from build123d import *

# Parameters (mm, degrees)
F0_W     = 72
F0_H     = 45
F1_DEPTH = 30
F3_DEPTH = 18
F4_R     = 2
F5_DEPTH = 19
F6_R     = 1.5
F7_R     = 3


with BuildPart() as f1:
    # F0 (on Front) → F1 (new body)
    with BuildSketch(Plane.XZ):
        with Locations((-36, 0)):
            Rectangle(F0_W, F0_H)
    extrude(amount=-F1_DEPTH)

    # F2 (on face) → F3 (join)
    with BuildSketch(Plane.XZ):
        Polygon((-64, 10.8), (-64, -10.8), (-57.15, -17.65), (-50.3, -10.8), (-50.3, 10.8), (-57.15, 17.65), align=None)
    extrude(amount=F3_DEPTH)

    # F4 (on face) → F5 (join)
    with BuildSketch(Plane.XZ.offset(18)):
        with Locations((-57.15, 9.3)):
            Circle(F4_R)
        with Locations((-57.15, -9.3)):
            Circle(F4_R)
    extrude(amount=F5_DEPTH)

    # F6
    f6_edges = [f1.edges().sort_by_distance(p)[0] for p in [
        (-59.15, -37, 9.3),
        (-59.15, -37, -9.3),
    ]]
    fillet(f6_edges, radius=F6_R)

    # F7
    f7_edges = [f1.edges().sort_by_distance(p)[0] for p in [
        (-72, 15, 22.5),
        (-72, 15, -22.5),
        (-72, 0, 0),
        (-72, 30, 0),
        (0, 15, -22.5),
        (0, 15, 22.5),
        (0, 0, 0),
        (0, 30, 0),
        (-36, 0, 22.5),
        (-36, 30, 22.5),
        (-36, 0, -22.5),
        (-36, 30, -22.5),
    ]]
    fillet(f7_edges, radius=F7_R)


solid = f1.part
Work out the finished part from the listing and answer in its coordinate system (mm). A direction names the side the tool comes from. Give positions to 0.01 mm unless a question says otherwise; leave off trailing zeros. Order: outer loops, then holes, each group sorted by start corner. A loop starts at its lowest first (then second) coordinate and runs counter-clockwise, first axis right, second up. Notation, with made-up numbers: (86, 10.5) - (101, 10.5) arc R22 ccw to (101, 40.5) - close; hole circle Ø4 at (63.25, 60). An arc over 180 degrees is marked (long way). Answer as CSV lines item,"result". Start each with the question number.
Q1. The mould has two halves that part along Z. Classify faces 5 (the face through (-59.148, -26.627, -9.212)), 6 (the face through (-57, -18, 0)), 7 (the face through (-36, 15, -22.5)), 8 (the face through (-64, -9, 0)): +Z half, -Z half, draft (parallel to the pull), parting line (faces both ways), or undercut.
Q2. Given pin 1 Ø5.5 at (y, z) = (-12, 1.5) entering from -X; pin 2 Ø3 at (y, z) = (-15.5, -16.5) entering from +X; pin 3 Ø12 at (y, z) = (-2, -4.5) entering from -X; pin 4 Ø8 at (y, z) = (-28.5, -13.5) entering from +X, each flat-ended and moving along its own axis, determine where each tip first touches the part or whether it passes through.
Q3. For faces 1 (the face through (-53.8, -8.9, -14.3)), 2 (the face through (-59.148, -26.627, 9.388)), 3 (the face through (-50.3, -9, 0)), 4 (the face through (-60.5, -8.9, 14.3)), determine the directions among +Z, -Z, +X, -X, +Y, -Y from which every point of the face is accessible in a straight line to the end or side of a thin tool.
Q4. Find the intervals of material crossed by L1, parallel to Y at x = -24.5, z = 1.5; L2, parallel to X at y = -8, z = -1.5; L3, parallel to Y at x = -62, z = 4, in increasing order. Write a range as [from, to].
Q5. The part is cut by section C-C (x = -46). Write down the section's boundary in (y, z), then the cut area to 3 significant figures.
Q6. The part is cut by section B-B (y = -2.5). Write down the section's boundary in (x, z).
Q7. The part is cut by section D-D (z = 1). Write down the section's boundary in (x, y), then the cut area to 3 significant figures.
Q8. The part is cut by section A-A (z = 14). Write down the section's boundary in (x, y), then the cut area to 3 significant figures.
Check result:
1,face 5,"undercut"
1,face 6,"undercut"
1,face 7,"-Z half"
1,face 8,"draft"
2,pin 1,"stops at x = -64"
2,pin 2,"stops at x = -54.5"
2,pin 3,"stops at x = -72"
2,pin 4,"stops at x = -55.16"
3,face 1,"-Z, +X, -Y"
3,face 2,"-Y"
3,face 3,"+Z, -Z, +X, -Y"
3,face 4,"+Z, -X, -Y"
4,L1,"y = [0, 30]"
4,L2,"x = [-64, -50.3]"
4,L3,"y = [-18, 30]"
5,outline,"(0, -19.5) arc R3 ccw to (3, -22.5) - (27, -22.5) arc R3 ccw to (30, -19.5) - (30, 19.5) arc R3 ccw to (27, 22.5) - (3, 22.5) arc R3 ccw to (0, 19.5) - close"
5,area,"1,340 mm²"
6,outline,"(-64, -10.8) - (-57.15, -17.65) - (-50.3, -10.8) - (-50.3, 10.8) - (-57.15, 17.65) - (-64, 10.8) - close"
7,outline,"(-72, 3) arc R3 ccw to (-69, 0) - (-64, 0) - (-64, -18) - (-50.3, -18) - (-50.3, 0) - (-3, 0) arc R3 ccw to (0, 3) - (0, 27) arc R3 ccw to (-3, 30) - (-69, 30) arc R3 ccw to (-72, 27) - close"
7,area,"2,400 mm²"
8,outline,"(-72, 3) arc R3 ccw to (-69, 0) - (-60.8, 0) - (-60.8, -18) - (-53.5, -18) - (-53.5, 0) - (-3, 0) arc R3 ccw to (0, 3) - (0, 27) arc R3 ccw to (-3, 30) - (-69, 30) arc R3 ccw to (-72, 27) - close"
8,area,"2,280 mm²"
